The drawing under review shows one solid part. Ordinate dimensions are in mm from its lowest x, y, z. Give positions to 0.01 mm unless a question says otherwise; leave off trailing zeros. Write each loop counter-clockwise with the first axis right and the second up, starting at its lowest first coordinate (ties: lowest second). Pieces come first, ordered by that corner, then holes. Notation, with made-up numbers: (-2.75, 78.25) -> (40.25, 78.25) arc R23 cw to (40.25, 87.25) -> close; hole circle Ø5 at (88.25, 38.5). An arc over 180 degrees is marked (long way). Write item = value, one per line.
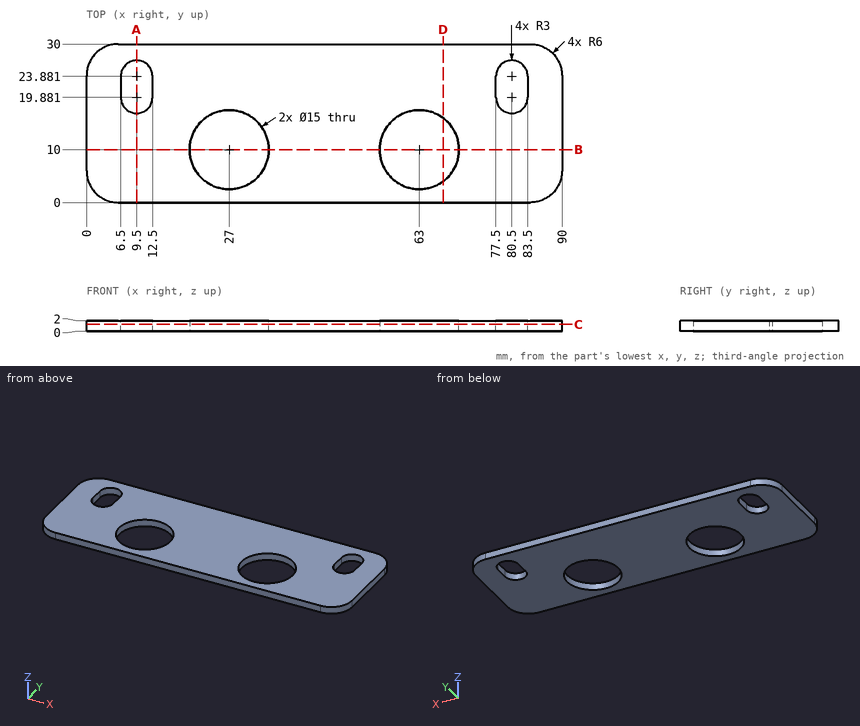
(1) Take a section at C-C (z = 1.25). Write out the cut boundary in (x, y), plus the area to 3 significant figures.
Answers below:
outline = (0, 6) arc R6 ccw to (6, 0) -> (84, 0) arc R6 ccw to (90, 6) -> (90, 24) arc R6 ccw to (84, 30) -> (6, 30) arc R6 ccw to (0, 24) -> close; hole (6.5, 19.88) arc R3 ccw to (12.5, 19.88) -> (12.5, 23.88) arc R3 ccw to (6.5, 23.88) -> close; hole circle Ø15 at (27, 10); hole circle Ø15 at (63, 10); hole (77.5, 19.88) arc R3 ccw to (83.5, 19.88) -> (83.5, 23.88) arc R3 ccw to (77.5, 23.88) -> close
area = 2,210 mm^2
(2) To check wall thickness, follow probe 1 along X at (y, z) = (10, 0.4); probe 2 along Y at (x, z) = (63, 1.4); probe 3 along X at (y, z) = (24.5, 1.2) (1 decimal). State the ranges of each line that lie inside material, in increasing order.
Answers below:
probe_1 = 0 to 19.5, 34.5 to 55.5, 70.5 to 90
probe_2 = 0 to 2.5, 17.5 to 30
probe_3 = 0 to 6.6, 12.4 to 77.6, 83.4 to 90
(3) Take a section at D-D (x = 67.5). Write out the cut boundary in (y, z), plus the area to 3 significant figures.
Answers below:
outline = (0, 0) -> (4, 0) -> (4, 2) -> (0, 2) -> close; (16, 0) -> (30, 0) -> (30, 2) -> (16, 2) -> close
area = 36.0 mm^2
(4) Take a section at B-B (y = 10). Write out the cut boundary in (x, z).
Answers below:
outline = (0, 0) -> (19.5, 0) -> (19.5, 2) -> (0, 2) -> close; (34.5, 0) -> (55.5, 0) -> (55.5, 2) -> (34.5, 2) -> close; (70.5, 0) -> (90, 0) -> (90, 2) -> (70.5, 2) -> close
(5) Take a section at A-A (x = 9.5). Write out the cut boundary in (y, z), plus the area to 3 significant figures.
Answers below:
outline = (0, 0) -> (16.88, 0) -> (16.88, 2) -> (0, 2) -> close; (26.88, 0) -> (30, 0) -> (30, 2) -> (26.88, 2) -> close
area = 40.0 mm^2
